Read the model definition and answer for the solid it produces. Units are mm, in the model's axes. Face numbers are marked on the shaded views. Coordinates: 2 decimals unless noted, no trailing zeros. Loops run counter-clockwise (first coordinate to the right, second up) from the corner with the lowest first, then second, coordinate; pieces in that order, holes last.
Q1. Straight lines are drawn through the part: line 1 (Z direction, x = 22, y = 64.5); line 2 (Y direction, x = 24.5, z = 64); line 3 (X direction, y = 234, z = -195). For each, find the intervals that lie inside material, in ascending order.
Q2. Section C-C (y = 51.5) is taken. Give the vertices of the cut face in (x, z), then the cut area to 3 significant figures.
Q3. A flat-ended cylindrical pin translates along its axis: P1, Ø3, axis at y = 96, z = 170.5, coming from the -X side. Find the tip coordinate at first contact, or state that the pin passes through.
Q4. Section B-B (z = 78.5) is taken. Give the vertices of the cut face in (x, y), then the cut area to 3 significant figures.
Q5. Section D-D (z = -79) is taken. Give the vertices of the cut face in (x, y), then the cut area to 3 significant figures.
Q6. The mould has two halves that part along Z. Classify the marked faces 1 and 2: pulls with the +Z half, pulls with the -Z half, needs draft (parallel to the pull), parting line crosses it, or undercut.
Q7. Section A-A (x = 10) is taken. Give the vertices of the cut face in (y, z).
from build123d import *

# Parameters (mm, degrees)
F0_W     = 895
F0_H     = 440
F1_DEPTH = 28
F2_T     = -2
F4_W     = 28
F4_H     = 200
F5_DEPTH = 2


with BuildPart() as f1:
    # F0 (on Right) → F1 (new body)
    with BuildSketch(Plane.YZ):
        Rectangle(F0_W, F0_H)
    extrude(amount=F1_DEPTH)

    # F2
    f2_openings = [f1.faces().sort_by_distance(p)[0] for p in [
        (0, 0, 0),
    ]]
    offset(amount=F2_T, openings=f2_openings)

    # F4 (on face) → F5 (join)
    with BuildSketch(Plane(origin=(0, 0, 0), x_dir=(0, -1, 0), z_dir=(-1, 0, 0))):
        with Locations((-433.5, -120)):
            Rectangle(F4_W, F4_H)
        with Locations((433.5, -120)):
            Rectangle(F4_W, F4_H)
    extrude(amount=-F5_DEPTH)


solid = f1.part
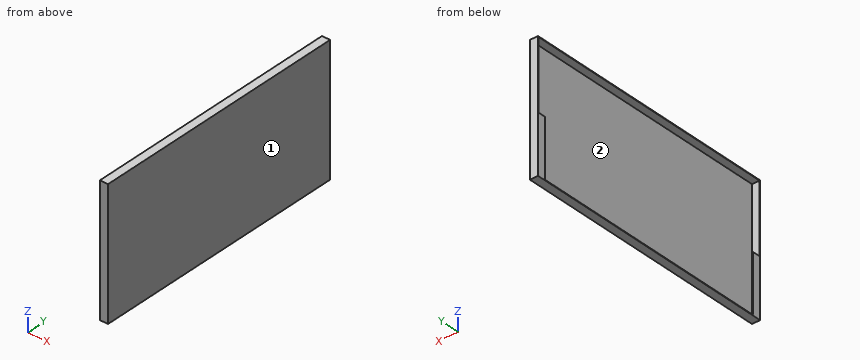
Numbers:
1. line 1: z = -220 to -218, 218 to 220
1. line 2: y = -447.5 to -445.5, 445.5 to 447.5
1. line 3: x = 26 to 28
2. outline: (0, -220) - (28, -220) - (28, 220) - (0, 220) - (0, 218) - (26, 218) - (26, -218) - (0, -218) - close
2. area: 984 mm2
3. P1: stops at x = 26
4. outline: (0, -447.5) - (28, -447.5) - (28, 447.5) - (0, 447.5) - (0, 445.5) - (26, 445.5) - (26, -445.5) - (0, -445.5) - close
4. area: 1,890 mm2
5. outline: (0, -447.5) - (28, -447.5) - (28, 447.5) - (0, 447.5) - (0, 419.5) - (2, 419.5) - (2, 445.5) - (26, 445.5) - (26, -445.5) - (2, -445.5) - (2, -419.5) - (0, -419.5) - close
5. area: 2,000 mm2
6. face 1: needs draft
6. face 2: undercut
7. outline: (-447.5, -220) - (447.5, -220) - (447.5, 220) - (-447.5, 220) - close; hole (-445.5, -218) - (445.5, -218) - (445.5, 218) - (-445.5, 218) - close
